from build123d import *

# Parameters (mm, degrees)
BOSS_EXTRUDE1_DEPTH = 3
FILLET3_R           = 3
SKETCH2_R           = 1.5
CUT_EXTRUDE1_DEPTH  = 72.126647608
SKETCH3_R           = 2.5
CUT_EXTRUDE2_DEPTH  = 1


with BuildPart() as part:
    # Sketch1 → Boss-Extrude1 (new body)
    with BuildSketch(Plane.XY):
        with BuildLine():
            Line((52, -45), (-52, -45))
            ThreePointArc((-52, -45), (-54.121320344, -44.121320344), (-55, -42))
            Line((-55, -42), (-55, 42))
            ThreePointArc((-55, 42), (-54.121320344, 44.121320344), (-52, 45))
            Line((-52, 45), (52, 45))
            ThreePointArc((52, 45), (54.121320344, 44.121320344), (55, 42))
            Line((55, 42), (55, -42))
            ThreePointArc((55, -42), (54.121320344, -44.121320344), (52, -45))
        make_face()
    extrude(amount=BOSS_EXTRUDE1_DEPTH)

    # Fillet3
    fillet3_edges = [part.edges().sort_by_distance(p)[0] for p in [
        (0, -45, 3),
        (-54.121320344, -44.121320344, 3),
        (-55, 0, 3),
        (-54.121320344, 44.121320344, 3),
        (0, 45, 3),
        (54.121320344, 44.121320344, 3),
        (55, 0, 3),
        (54.121320344, -44.121320344, 3),
    ]]
    fillet(fillet3_edges, radius=FILLET3_R - 0.0001)  # a hair under: the kernel refuses the full size

    # Sketch2 → Cut-Extrude1 (cut, through all)
    with BuildSketch(Plane.XY.offset(3)):
        with Locations((-50.25, 40.25)):
            Circle(SKETCH2_R)
        with Locations((50.25, 40.25)):
            Circle(SKETCH2_R)
        with Locations((-50.25, -40.25)):
            Circle(SKETCH2_R)
        with Locations((50.25, -40.25)):
            Circle(SKETCH2_R)
    extrude(amount=-CUT_EXTRUDE1_DEPTH, mode=Mode.SUBTRACT)

    # Sketch3 → Cut-Extrude2 (cut)
    with BuildSketch(Plane.XY.offset(3)):
        with Locations((-50.25, 40.25)):
            Circle(SKETCH3_R)
        with Locations((50.25, 40.25)):
            Circle(SKETCH3_R)
        with Locations((-50.25, -40.25)):
            Circle(SKETCH3_R)
        with Locations((50.25, -40.25)):
            Circle(SKETCH3_R)
    extrude(amount=-CUT_EXTRUDE2_DEPTH, mode=Mode.SUBTRACT)


solid = part.part
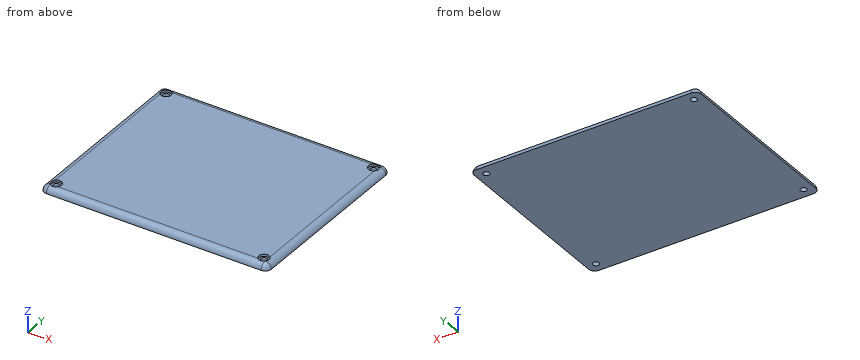
Geometry check sheet. Reference: the model listing, model coordinates, mm. Give positions to 0.01 mm unless a question says otherwise; leave off trailing zeros.
(1) Thickness scan on L1, parallel to Y at x = 50.25, z = 2.6; L2, parallel to Y at x = -49, z = 1.25; L3, parallel to X at y = -38.5, z = 2.55. Record the ranges inside material, lowest first.
From the geometry:
L1: y = -43.5 to -42.75, -37.75 to 37.75, 42.75 to 43.5
L2: y = -44.73 to -41.08, -39.42 to 39.42, 41.08 to 44.73
L3: x = -53.58 to -52.04, -48.46 to 48.46, 52.04 to 53.58
(2) Section check A-A on y = -40.25. Count the separate pieces of the cut face and the enclosed holes in it, then the cut area to 3 significant figures.
From the geometry:
separate pieces: 3
enclosed holes: 0
area: 304 mm2
(3) Depth check by flat-ended pin: pin 1 Ø5 at (x, y) = (-50.25, -40.25) entering from -Z; pin 2 Ø2.5 at (x, y) = (-50, -40) entering from +Z; pin 3 Ø1.5 at (y, z) = (-18.5, 1) entering from +X; pin 4 Ø1.8 at (x, y) = (50.25, 40.25) entering from +Z. Enter the tip coordinate at first touch or a pass-through.
From the geometry:
pin 1: stops at z = 0
pin 2: stops at z = 2
pin 3: stops at x = 54.99
pin 4: passes through
